Geometry check sheet. Reference: the model listing, model coordinates, mm. Round coordinates to 2 decimals unless told otherwise and drop trailing zeros. Loops run counter-clockwise (first coordinate to the right, second up) from the corner with the lowest first, then second, coordinate; pieces in that order, holes last. Notation, with made-up numbers: (-28, 67) - (23, 67) arc R22 ccw to (23, 80) - close; hole circle Ø5 at (72.25, 62.25). An arc over 180 degrees is marked (long way). Answer as CSV lines item,"result". Start each with the question number.
1) Cross-section at B-B on x = 3.5. Record the boundary of the cut face in (y, z), and give its area (3 significant figures).
2) Cross-section at C-C on z = 0.25. State how many separate pieces and enclosed holes the cut face has, and give its area (3 significant figures).
3) Cross-section at A-A on y = -5. Record the boundary of the cut face in (x, z), and give its area (3 significant figures).
4) Thickness scan on line 1 along Y through (x, z) = (-3.5, 0.35); line 2 along Y through (x, z) = (-10.75, 0.4); line 3 along X through (y, z) = (6, -0.6). Record the ranges inside material, lowest first.
from build123d import *

# Parameters (mm, degrees)
BOSS_EXTRUDE1_DEPTH = 0.8
SKETCH4_R           = 1.6
CUT_EXTRUDE3_DEPTH  = 22.346779617
SKETCH5_R           = 1.2
CUT_EXTRUDE4_DEPTH  = 22.346779617


with BuildPart() as part:
    # Sketch1 → Boss-Extrude1 (new, symmetric)
    with BuildSketch(Plane.XY):
        with BuildLine():
            Line((-13.75, 13.25), (-13.75, -13.25))
            ThreePointArc((-13.75, -13.25), (-12.871320344, -15.371320344), (-10.75, -16.25))
            Line((-10.75, -16.25), (10.75, -16.25))
            ThreePointArc((10.75, -16.25), (12.871320344, -15.371320344), (13.75, -13.25))
            Line((13.75, -13.25), (13.75, 13.25))
            ThreePointArc((13.75, 13.25), (12.871320344, 15.371320344), (10.75, 16.25))
            Line((10.75, 16.25), (-10.75, 16.25))
            ThreePointArc((-10.75, 16.25), (-12.871320344, 15.371320344), (-13.75, 13.25))
        make_face()
    extrude(amount=BOSS_EXTRUDE1_DEPTH, both=True)

    # Sketch4 → Cut-Extrude3 (cut, through all)
    with BuildSketch(Plane.XY.offset(0.8)):
        with Locations((10.75, 13.25)):
            Circle(SKETCH4_R)
        with Locations((10.75, -13.25)):
            Circle(SKETCH4_R)
        with Locations((-10.75, -13.25)):
            Circle(SKETCH4_R)
        with Locations((-10.75, 13.25)):
            Circle(SKETCH4_R)
    extrude(amount=-CUT_EXTRUDE3_DEPTH, mode=Mode.SUBTRACT)

    # Sketch5 → Cut-Extrude4 (cut, through all)
    with BuildSketch(Plane.XY.offset(0.8)):
        with Locations((3.5, -5)):
            Circle(SKETCH5_R)
        with Locations((0, -5)):
            Circle(SKETCH5_R)
        with Locations((-3.5, -5)):
            Circle(SKETCH5_R)
        with Locations((3.5, 5)):
            Circle(SKETCH5_R)
        with Locations((0, 5)):
            Circle(SKETCH5_R)
        with Locations((-3.5, 5)):
            Circle(SKETCH5_R)
        with Locations((-3.5, 0)):
            Circle(SKETCH5_R)
        Circle(SKETCH5_R)
        with Locations((3.5, 0)):
            Circle(SKETCH5_R)
    extrude(amount=-CUT_EXTRUDE4_DEPTH, mode=Mode.SUBTRACT)


solid = part.part
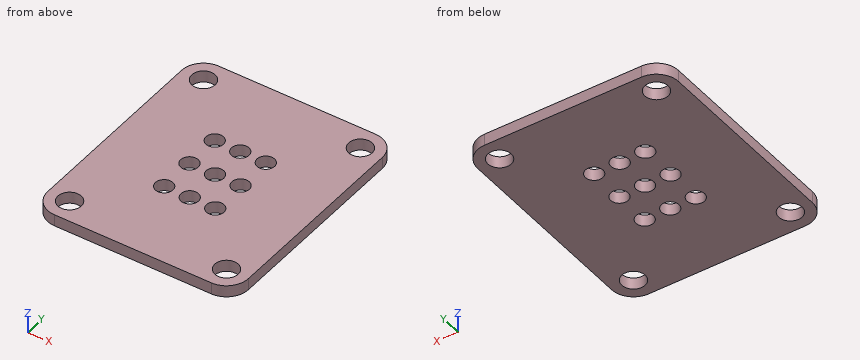
Answer block:
1,outline,"(-16.25, -0.8) - (-6.2, -0.8) - (-6.2, 0.8) - (-16.25, 0.8) - close; (-3.8, -0.8) - (-1.2, -0.8) - (-1.2, 0.8) - (-3.8, 0.8) - close; (1.2, -0.8) - (3.8, -0.8) - (3.8, 0.8) - (1.2, 0.8) - close; (6.2, -0.8) - (16.25, -0.8) - (16.25, 0.8) - (6.2, 0.8) - close"
1,area,"40.5 mm^2"
2,separate pieces,"1"
2,enclosed holes,"13"
2,area,"813 mm^2"
3,outline,"(-13.75, -0.8) - (-4.7, -0.8) - (-4.7, 0.8) - (-13.75, 0.8) - close; (-2.3, -0.8) - (-1.2, -0.8) - (-1.2, 0.8) - (-2.3, 0.8) - close; (1.2, -0.8) - (2.3, -0.8) - (2.3, 0.8) - (1.2, 0.8) - close; (4.7, -0.8) - (13.75, -0.8) - (13.75, 0.8) - (4.7, 0.8) - close"
3,area,"32.5 mm^2"
4,line 1,"y = -16.25 to -6.2, -3.8 to -1.2, 1.2 to 3.8, 6.2 to 16.25"
4,line 2,"y = -16.25 to -14.85, -11.65 to 11.65, 14.85 to 16.25"
4,line 3,"x = -13.75 to -4.16, -2.84 to -0.66, 0.66 to 2.84, 4.16 to 13.75"
